Geometry: final body of the model. Coordinates: model frame, mm. A direction names the side the tool comes from. Give positions to 0.01 mm unless a question says otherwise; leave off trailing zeros. Order: outer loops, then holes, each group sorted by start corner. A loop starts at its lowest first (then second) coordinate and runs counter-clockwise, first axis right, second up. Notation, with made-up numbers: (-34, -4.5) -> (15, -4.5) arc R28 cw to (15, 21.5) -> close; hole circle Ø9 at (71, 82.25). An arc over 180 degrees is marked (long way). Answer in a Markdown table with one row per item. Add a question column.
Q1. Cut plane C-C on x = 13. Return the cut outline in (y, z).
Q2. Cut plane A-A on x = 7.5. Return the cut outline in (y, z), and give its area (3 significant figures).
Q3. Contact query for flat-ended pins moving along their axis: P1, Ø1, axis at y = 1, z = 14.5, coming from the -X side; P2, Ø5.5, axis at y = -5.5, z = 29.5, coming from the +X side; P3, Ø6, axis at y = -2.5, z = 18, coming from the +X side; P4, Ø5, axis at y = -3.5, z = 15, coming from the -X side. Output: stop coordinate, or through.
Q4. Cut plane D-D on z = 26.5. Return the cut outline in (x, y), and give its area (3 significant figures).
Q5. Set-up query: faces 5 (the face through (0, -4, 30)), 6 (the face through (-2.4, 2.3, 34.3)), 7 (the face through (-0.5, -4.5, 34.5)). Return all of +Z, -Z, +X, -X, +Y, -Y with unobstructed straight access to the full face (end or side cutting, diameter ignored); none if empty.
Q6. Pull-direction query (Z, two-part tool) for faces 1 (the face through (6.35, 1.49, 12.77)), 2 (the face through (0.5, 1.2, 0.5)), 3 (the face through (-0.7, -8.4, 34.3)), 4 (the face through (14.5, 0.5, 17.3)); classes: +Z half, -Z half, draft (parallel to the pull), parting line (faces both ways), or undercut.
Q7. Cut plane B-B on z = 10. Return the cut outline in (x, y).
Q8. Line query: line 1 along X through (y, z) = (1.3, 10); line 2 along Y through (x, z) = (7, 22); line 3 along X through (y, z) = (-3.25, 32.5). Output: solid intervals per line, ascending. Write a range as from..to.
from build123d import *

# Parameters (mm, degrees)
SKETCH_1_W           = 15
SKETCH_1_H           = 20
SKETCH_1_R           = 3
EXTRUDE_1_DEPTH      = 3
SKETCH_2_W           = 15
SKETCH_2_H           = 15
EXTRUDE_2_DEPTH      = 3
EXTRUDE_3_DEPTH      = 9
EXTRUDE_3_DEPTH_BACK = 3
SKETCH_4_W           = 3
SKETCH_4_H           = 8
CHAMFER_1_SIZE       = 1


with BuildPart() as part:
    # 草图1 → 凸台-拉伸1 (new body)
    with BuildSketch(Plane(origin=(0, 0, 0), x_dir=(1, 0, 0), z_dir=(0, 1, 0))):
        with Locations((7.5, -10)):
            Rectangle(SKETCH_1_W, SKETCH_1_H)
        with Locations(Location((7.5, -10, 0), (0, 0, 270))):
            Circle(SKETCH_1_R, mode=Mode.SUBTRACT)
    extrude(amount=EXTRUDE_1_DEPTH)

    # 草图2 → 凸台-拉伸2 (add)
    with BuildSketch(Plane(origin=(0, 3, 0), x_dir=(1, 0, 0), z_dir=(0, 1, 0))):
        with Locations((7.5, -27.5)):
            Rectangle(SKETCH_2_W, SKETCH_2_H)
    extrude(amount=-EXTRUDE_2_DEPTH)

    # 草图4 → 凸台-拉伸3 (add, two sides: drawn at the far end of the back side and taken through both)
    with BuildSketch(Plane.XZ.offset(-EXTRUDE_3_DEPTH_BACK)):
        with Locations((-1.5, 31)):
            Rectangle(SKETCH_4_W, SKETCH_4_H)
    extrude(amount=EXTRUDE_3_DEPTH + EXTRUDE_3_DEPTH_BACK)

    # 倒角1
    chamfer_1_edges = [part.edges().sort_by_distance(p)[0] for p in [
        (7.5, 0, 7),
        (7.5, 3, 7),
        (15, 3, 17.5),
        (7.5, 3, 0),
        (7.5, 0, 35),
        (15, 1.5, 35),
        (6, 3, 35),
        (0, 0, 31),
        (0, -4.5, 35),
        (-1.5, 3, 27),
        (-3, -3, 27),
        (-3, 3, 31),
        (-3, -3, 35),
        (0, -9, 31),
        (-1.5, -9, 35),
        (-3, -9, 31),
        (0, 3, 13.5),
        (7.5, 0, 0),
        (15, 0, 17.5),
        (0, 1.5, 0),
        (15, 1.5, 0),
    ]]
    chamfer(chamfer_1_edges, length=CHAMFER_1_SIZE)


solid = part.part
Completed:
| question | item | result |
|---|---|---|
| 1 | outline | (0, 1) -> (1, 0) -> (2, 0) -> (3, 1) -> (3, 34) -> (2, 35) -> (1, 35) -> (0, 34) -> close |
| 2 | outline | (0, 1) -> (1, 0) -> (2, 0) -> (3, 1) -> (3, 6) -> (2, 7) -> (1, 7) -> (0, 6) -> close; (0, 14) -> (1, 13) -> (2, 13) -> (3, 14) -> (3, 34) -> (2, 35) -> (1, 35) -> (0, 34) -> close |
| 2 | area | 83.0 mm² |
| 3 | P1 | stops at x = 0 |
| 3 | P2 | stops at x = 0 |
| 3 | P3 | stops at x = 14.5 |
| 3 | P4 | passes through |
| 4 | outline | (0, 0) -> (14, 0) -> (15, 1) -> (15, 2) -> (14, 3) -> (1, 3) -> (0, 2) -> close |
| 4 | area | 43.5 mm² |
| 5 | face 5 | +Z, -Z, +X, -Y |
| 5 | face 6 | +Z, -X, +Y |
| 5 | face 7 | +Z, +X, -Y |
| 6 | face 1 | undercut |
| 6 | face 2 | -Z half |
| 6 | face 3 | +Z half |
| 6 | face 4 | draft |
| 7 | outline | (0, 0) -> (3.5, 0) -> (4.5, 1) -> (4.5, 2) -> (3.5, 3) -> (1, 3) -> (0, 2) -> close; (10.5, 1) -> (11.5, 0) -> (14, 0) -> (15, 1) -> (15, 2) -> (14, 3) -> (11.5, 3) -> (10.5, 2) -> close |
| 8 | line 1 | x = 0..4.5, 10.5..15 |
| 8 | line 2 | y = 0..3 |
| 8 | line 3 | x = -3..0 |
